Autodesk Fusion 360 part; units mm, degrees
sketch "Boceto1" plane through (0, 0, 0) normal (1, 0, 0) x (0, 1, 0)
sketch "Boceto2" plane through (0, 0, 0) normal (1, 0, 0) x (0, 1, 0)
  line L0 (-50, 0) -> (-35, 0)
  line L1 (35, 0) -> (50, 0)
  arc A0 (50, 0) -> (-50, 0) centre (0, 0) ccw
  arc A1 (35, 0) -> (-35, 0) centre (0, 0) ccw
  dimension "d1" = 100
  dimension "d2" = 15
extrude "Extruir1" add sketch "Boceto2" along normal blind 200
ref_plane "PlanoDeObra1" through (100, 0, 50) normal (0, 0, 1) x (0, -1, 0)
sketch "Boceto3" plane through (100, 0, 50) normal (0, 0, 1) x (1, 0, 0)
  line L0 (75, -15) -> (-75, -15)
  line L1 (-75, -15) -> (-75, 15)
  line L2 (-75, 15) -> (75, 15)
  line L3 (75, 15) -> (75, -15)
  line L4 (75, -15) -> (-75, 15) construction
  line L5 (-75, -15) -> (75, 15) construction
  dimension "d6" = 150
  dimension "d7" = 30
extrude "Extruir2" cut sketch "Boceto3" along normal up to surface end surface at (66.6667, -26.8116, 22.4976)
sketch "Boceto4" plane through (0, 0, 0) normal (0, 0, 1) x (1, 0, 0)
Work out the finished part from the listing and answer in its coordinate system (mm). A direction names the side the tool comes from. Give positions to 0.01 mm unless a question says otherwise; leave off trailing zeros. Order: outer loops, then holes, each group sorted by start corner. A loop starts at its lowest first (then second) coordinate and runs counter-clockwise, first axis right, second up. Notation, with made-up numbers: (33, 38.25) -> (54, 38.25) arc R31 cw to (54, 66.25) -> close; hole circle Ø6 at (-37.75, -27). An arc over 180 degrees is marked (long way). One line per item, written item: value.
Item 1: Determine the mould class of faces 3 (the flat face through (0, -1, 36)), 4 (the flat face through (200, -1, 36)), 5 (the flat face through (99, -43, 0)), 6 (the flat face through (25, 0, 41)) for opening direction X: released by +X, released by -X, zero draft, split by the parting line, or undercut.
Answer sheet:
face 3: released by -X
face 4: released by +X
face 5: zero draft
face 6: undercut
Item 2: Find section B-B, the plane y = 0. Give the vertices of the cut face in (x, z), plus the area to 3 significant figures.
Answer sheet:
outline: (0, 35) -> (25, 35) -> (25, 50) -> (0, 50) -> close; (175, 35) -> (200, 35) -> (200, 50) -> (175, 50) -> close
area: 750 mm²
Item 3: Find section D-D, the plane x = 185. Give the vertices of the cut face in (y, z).
Answer sheet:
outline: (-50, 0) -> (-35, 0) arc R35 cw to (35, 0) -> (50, 0) arc R50 ccw to start
Item 4: Flat-ended cylindrical pins translate along their axes: P1, Ø4, axis at x = 178.5, z = 25, coming from the +Y side; P2, Ø17.5, axis at x = 106, z = 43.5, coming from the +Y side; P3, Ø12, axis at y = 5, z = 33, coming from the -X side; P4, Ø5, axis at x = 109, z = 44.5, coming from the -Y side. Find the tip coordinate at first contact, or state that the pin passes through.
Answer sheet:
P1: y = 44.4
P2: y = 35.95
P3: x = 0
P4: y = -27.13
Item 5: Find section C-C, the plane z = 42. Give the vertices of the cut face in (x, y).
Answer sheet:
outline: (0, -27.13) -> (200, -27.13) -> (200, 27.13) -> (0, 27.13) -> close; hole (25, -15) -> (175, -15) -> (175, 15) -> (25, 15) -> close
Item 6: Straight lines are drawn through the part: probe 1 along X at (y, z) = (13, 42.5); probe 2 along Y at (x, z) = (53.5, 2.5); probe 3 along Y at (x, z) = (53, 15). For each, find the intervals that lie inside material, in ascending order.
Answer sheet:
probe 1: 0 to 25, 175 to 200
probe 2: -49.94 to -34.91, 34.91 to 49.94
probe 3: -47.7 to -31.62, 31.62 to 47.7
Item 7: A tool of negligible diameter and unlimited length cuts with its end or side. For faces 1 (the cylindrical face through (98.6, -23.08, 26.31)), 2 (the flat face through (175, 0, 41)), from which of +Z, -Z, +X, -X, +Y, -Y can it reach the whole face along a straight path? Write none if from no direction.
Answer sheet:
face 1: -Z, +X, -X
face 2: +Z, -Z
Item 8: Find section A-A, the plane x = 51. Give the vertices of the cut face in (y, z), plus the area to 3 significant figures.
Answer sheet:
outline: (-50, 0) -> (-35, 0) arc R35 cw to (-15, 31.62) -> (-15, 47.7) arc R50 ccw to start; (15, 31.62) arc R35 cw to (35, 0) -> (50, 0) arc R50 ccw to (15, 47.7) -> close
area: 1,540 mm²
